Here's the drawing with two shaded views (mm, measured from the low corner). I have some questions. A direction names the side the tool comes from. Give positions to 0.01 mm unless a question says otherwise; leave off trailing zeros. Write each loop counter-clockwise with the first axis right and the second up, starting at its lowest first coordinate (ties: lowest second). Pieces come first, ordered by that corner, then holes.
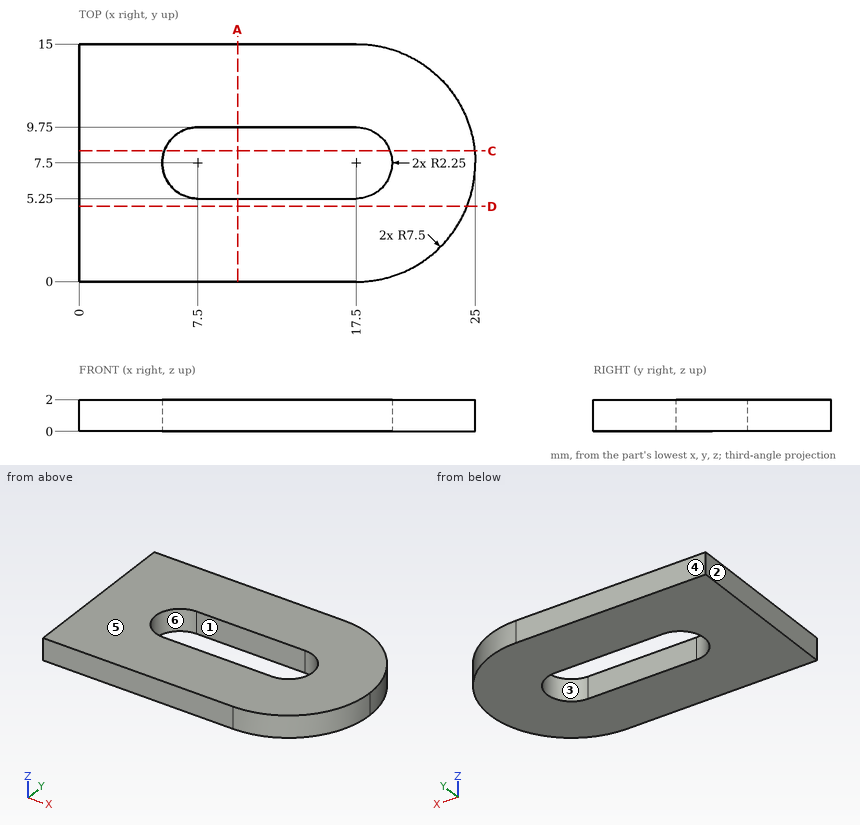
(1) Imagine slicing it at D-D, the plane y = 4.75. Write out the boundary of the cut face in (x, z).
Returned:
outline: (0, 0) - (24.48, 0) - (24.48, 2) - (0, 2) - close
(2) If we mould it in two halves opening along X, with no side actions, what happens to the marked faces 1, 2, 3 and 4? For each: +X half, -X half, draft (parallel to the pull), parting line (faces both ways), or undercut.
Returned:
face 1: undercut
face 2: -X half
face 3: undercut
face 4: draft
(3) Imagine slicing it at A-A, the plane x = 10. Write out the boundary of the cut face in (y, z).
Returned:
outline: (0, 0) - (5.25, 0) - (5.25, 2) - (0, 2) - close; (9.75, 0) - (15, 0) - (15, 2) - (9.75, 2) - close
(4) If I drill on L1, parallel to Y at x = 9.5, z = 1.7; L2, parallel to X at y = 5.75, z = 1.85 (1 decimal); L3, parallel to Y at x = 18, z = 1.85 (1 decimal), over which ranges is the centre line in solid material (lowest first)?
Returned:
L1: y = 0 to 5.25, 9.75 to 15
L2: x = 0 to 6.1, 18.9 to 24.8
L3: y = 0 to 5.3, 9.7 to 15
(5) For the marked faces 5 and 6, which set-ups out of +Z, -Z, +X, -X, +Y, -Y let a thin tool reach every point of the face, with its end or its side?
Returned:
face 5: +Z, +X, -X, +Y, -Y
face 6: +Z, -Z
(6) Will this pin go through, and if not, where does the flat tip stop? P1, Ø6, axis at x = 21, y = 3.5, coming from the -Z side.
Returned:
P1: stops at z = 0
(7) Imagine slicing it at C-C, the plane y = 8.25. Write out the boundary of the cut face in (x, z).
Returned:
outline: (0, 0) - (5.38, 0) - (5.38, 2) - (0, 2) - close; (19.62, 0) - (24.96, 0) - (24.96, 2) - (19.62, 2) - close
